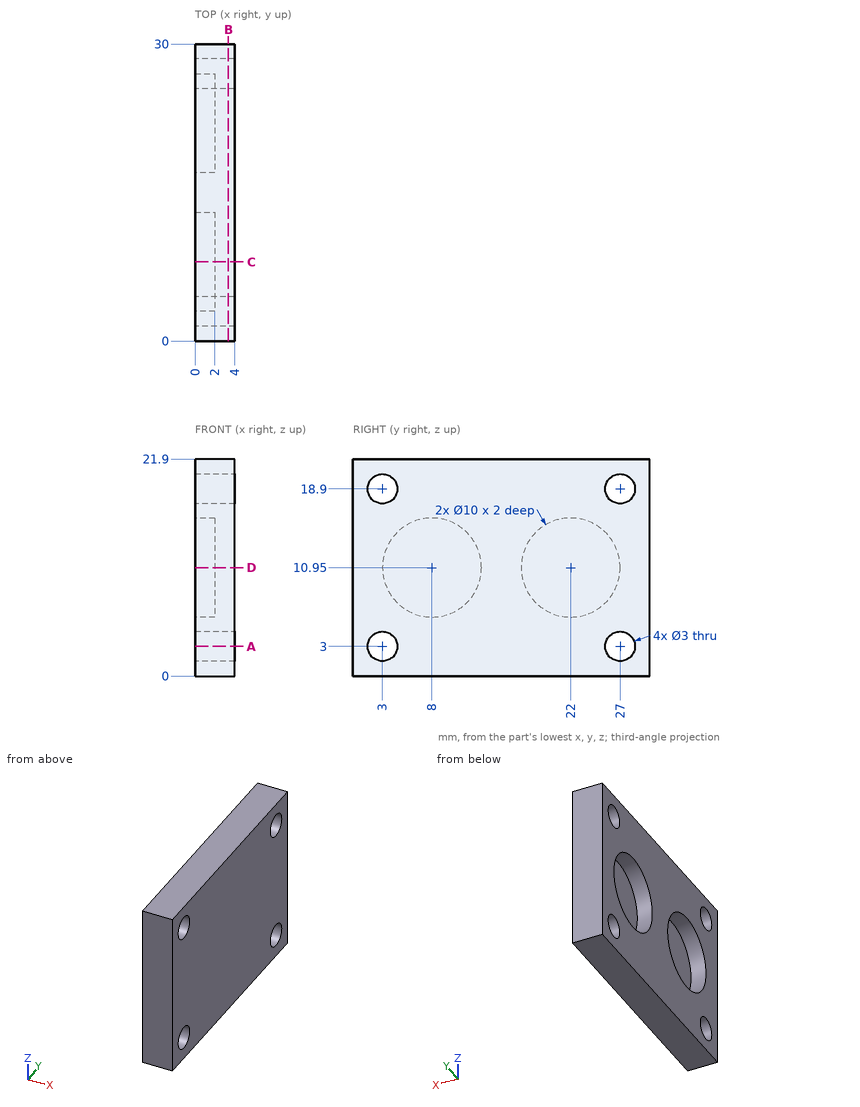
Could you check a few things on this drawing? It's one solid part, dimensions in mm from its lowest x, y, z. Round coordinates to 2 decimals unless told otherwise and drop trailing zeros. Order: outer loops, then holes, each group sorted by start corner. A loop starts at its lowest first (then second) coordinate and runs counter-clockwise, first axis right, second up. Notation, with made-up numbers: M -3,80 L 13,80 A21 cw 13,100 Z; hole C -28,7.25 d5. An arc over 180 degrees is marked long. One line per item, written item: value.
(1) Imagine slicing it at A-A (z = 3). Write out the boundary of the cut face in (x, y).
Ans:
outline: M 0,0 L 4,0 L 4,1.5 L 0,1.5 Z; M 0,4.5 L 4,4.5 L 4,25.5 L 0,25.5 Z; M 0,28.5 L 4,28.5 L 4,30 L 0,30 Z
(2) Imagine slicing it at D-D (z = 10.95). Write out the boundary of the cut face in (x, y).
Ans:
outline: M 0,0 L 4,0 L 4,30 L 0,30 L 0,27 L 2,27 L 2,17 L 0,17 L 0,13 L 2,13 L 2,3 L 0,3 Z
(3) Imagine slicing it at B-B (x = 3.35). Write out the boundary of the cut face in (y, z).
Ans:
outline: M 0,0 L 30,0 L 30,21.9 L 0,21.9 Z; hole C 3,3 d3; hole C 3,18.9 d3; hole C 27,3 d3; hole C 27,18.9 d3
(4) I'm going to push flat-ended pins straight in: P1, Ø1.5, axis at y = 9, z = 11.5, coming from the -X side; P2, Ø1.8, axis at y = 3, z = 3, coming from the -X side. Where does each tip first touch, or does it pass through?
Ans:
P1: stops at x = 2
P2: passes through
(5) Imagine slicing it at C-C (y = 8). Write out the boundary of the cut face in (x, z).
Ans:
outline: M 0,0 L 4,0 L 4,21.9 L 0,21.9 L 0,15.95 L 2,15.95 L 2,5.95 L 0,5.95 Z
(6) I need wall thicknesses on line 1 along Y through (x, z) = (1.3, 13.5); line 2 along Z through (x, y) = (3, 1.75); line 3 along Y through (x, z) = (2.3, 3). Which ranges of each line are inside material? Lowest first, please. Write a range as from..to.
Ans:
line 1: y = 0..3.7, 12.3..17.7, 26.3..30
line 2: z = 0..2.17, 3.83..18.07, 19.73..21.9
line 3: y = 0..1.5, 4.5..25.5, 28.5..30
